The model under review builds one solid part; all positions refer to its coordinate system, in mm. Face numbers are marked on the shaded views. A direction names the side the tool comes from. Give positions to 0.01 mm unless a question says otherwise; leave off trailing zeros. Order: outer loops, then holes, each group sorted by start corner. A loop starts at its lowest first (then second) coordinate and runs counter-clockwise, first axis right, second up. Notation, with made-up numbers: (7.25, 52) - (44.25, 52) arc R25 ccw to (44.25, 66) - close; hole circle Ø6 at (81.5, -12.75). An arc over 180 degrees is marked (long way). Answer as CSV lines item,"result". Start each with the question number.
from build123d import *

# Parameters (mm, degrees)
F2_DEPTH = 8
F4_R     = 5
F5_R     = 3.49999
F3_R     = 1.625
F8_DEPTH = 7.001


# Not quite as in the source:
# - a fillet or chamfer is up to 0.001 mm smaller than in the source, because OpenCascade refuses the exact size


with BuildPart() as f2:
    # F1 (on Top) → F2 (new body)
    with BuildSketch(Plane.XY):
        with BuildLine():
            Line((0, 7), (-17.4501655647, 7))
            ThreePointArc((-17.4501655647, 7), (-27.535987639, 9.7036800538), (-35.3366188286, 2.7622215766))
            Line((-35.3366188286, 2.7622215766), (-28.7587704831, 0.3680805733))
            ThreePointArc((-28.7587704831, 0.3680805733), (-24.8073034208, 2.9953558075), (-21.1270166538, 0))
            Line((-21.1270166538, 0), (0, 0))
            Line((0, 0), (0, 7))
        make_face()
    extrude(amount=F2_DEPTH)

    # F4
    f4_edges = [f2.edges().sort_by_distance(p)[0] for p in [
        (-17.450166, 7, 4),
        (-21.127017, 0, 4),
    ]]
    fillet(f4_edges, radius=F4_R)

    # F5 (radius 3.5 in the source; OpenCascade refuses exactly that, so slightly less here)
    f5_edges = [f2.edges().sort_by_distance(p)[0] for p in [
        (-35.336619, 2.762222, 4),
        (-28.75877, 0.368081, 4),
    ]]
    fillet(f5_edges, radius=F5_R)

    # F7: F2 across face


with BuildPart() as f2_1:
    add(f2.part)
    add(f2.part.mirror(Plane(origin=(0, 3.5, 4), x_dir=(0, 1, 0), z_dir=(1, 0, 0))))

    # F3 (on face) → F8 (cut, through all)
    with BuildSketch(Plane(origin=(0, 7, 0), x_dir=(-1, 0, 0), z_dir=(0, 1, 0))):
        with Locations((9.4501655647, 4)):
            Circle(F3_R)
    extrude(amount=-F8_DEPTH, mode=Mode.SUBTRACT)


solid = f2_1.part
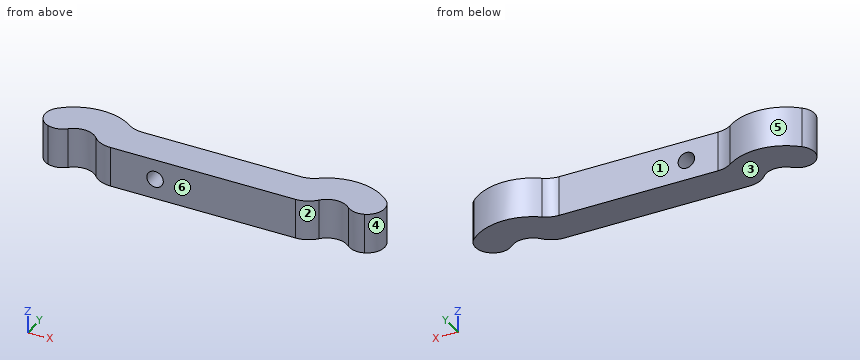
Item 1: For line 1 along Y through (x, z) = (-10, 0.75); line 2 along Z through (x, y) = (-9.5, 2.75); line 3 along X through (y, z) = (8.5, 5), list the stretches that pass through material, from the lowest coordinate up.
Item 2: Clearance check with flat-ended pins moving along their axes: pin 1 (4 mm diameter, centred on x = 1.5, z = 3.5, fed in from +Y); pin 2 (1.5 mm diameter, centred on x = 21.5, z = 3, fed in from +Y); pin 3 (2 mm diameter, centred on y = 1, z = 5, fed in from +X). State where each tip first meets the part, or that it passes through.
Item 3: Take a section at B-B on y = 9. Write out the cut boundary in (x, z), and give its area (3 significant figures).
Item 4: Mouldability with a two-part tool opening along X and no side actions: class the marked faces 4, 5 and 6 as released by +X, released by -X, zero draft, split by the parting line, or undercut.
Item 5: Machinability: for the marked faces 1, 2 and 3, which of the approach directions +Z, -Z, +X, -X, +Y, -Y give a long, thin tool a straight path to every point of the face, cutting with its end or side? Answer none if there is none.
Item 6: Take a section at D-D on y = 4.75. Write out the cut boundary in (x, z) (3 decimals), and give its area (3 significant figures).
Data:
1,line 1,"y = 0 to 7"
1,line 2,"z = 0 to 2.38, 5.62 to 8"
1,line 3,"x = -30.55 to -19.45, 19.45 to 30.55"
2,pin 1,"stops at y = 7"
2,pin 2,"stops at y = 9.65"
2,pin 3,"stops at x = 32.43"
3,outline,"(-29.58, 0) - (-20.42, 0) - (-20.42, 8) - (-29.58, 8) - close; (20.42, 0) - (29.58, 0) - (29.58, 8) - (20.42, 8) - close"
3,area,"147 mm^2"
4,face 4,"released by +X"
4,face 5,"undercut"
4,face 6,"zero draft"
5,face 1,"+Z, -Z, +Y"
5,face 2,"+Z, -Z, -Y"
5,face 3,"-Z, +X, -X, +Y, -Y"
6,outline,"(-33.531, 0) - (33.531, 0) - (33.531, 8) - (-33.531, 8) - close; hole circle Ø3.25 at (-9.45, 4)"
6,area,"528 mm^2"
